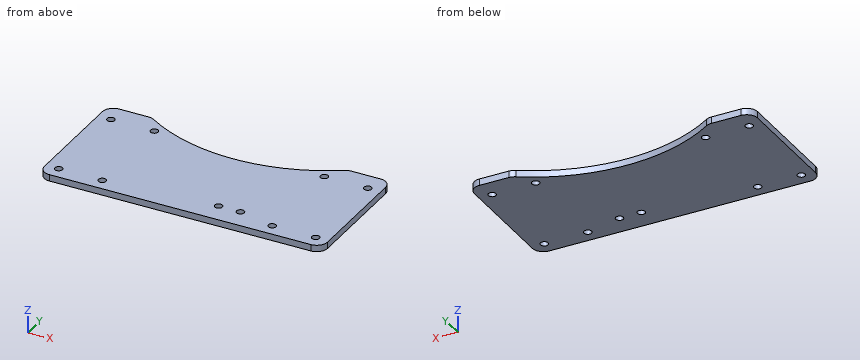
Autodesk Inventor part; units mm, degrees
ref_plane "YZ Plane" through (0, 0, 0) normal (1, 0, 0) x (0, 1, 0)
ref_plane "XZ Plane" through (0, 0, 0) normal (0, 1, 0) x (-1, 0, 0)
ref_plane "XY Plane" through (0, 0, 0) normal (0, 0, 1) x (1, 0, 0)
sketch "Sketch1" plane through (0, 0, 0) normal (0, 0, 1) x (1, 0, 0)
  line L0 (-65, -30) -> (65, -30)
  line L1 (65, -30) -> (65, 30)
  line L2 (65, 30) -> (-65, 30)
  line L3 (-65, 30) -> (-65, -30)
  line L4 (-65, -30) -> (65, 30) construction
  line L5 (65, -30) -> (-65, 30) construction
  arc A0 (-45, 30) -> (45, 30) centre (0, 96.6789) ccw
  point P0 (0, 0)
  dimension "d0" = 130
  dimension "d1" = 60
  dimension "d5" = 20
  dimension "d6" = 20
extrude "Extrusion1" add sketch "Sketch1" along normal blind 3 contours L3 L2 A0 L1 L0
fillet "Fillet1" radius 5 6 edges at (65, 30, 1.5) (65, -30, 1.5) (-65, -30, 1.5) (-65, 30, 1.5) (45, 30, 1.5) (-45, 30, 1.5)
sketch "Sketch2" plane through (0, 0, 3) normal (0, 0, 1) x (1, 0, 0)
  circle A0 centre (59, -24) radius 1.75
  circle A1 centre (39, -24) radius 1.75
  line L0 (65, -25) -> (65, 25)
  line L1 (-60, -30) -> (60, -30)
  circle A2 centre (59, 21) radius 1.75
  circle A3 centre (39, 21) radius 1.75
  line L2 (0, -30) -> (0, -45.4947)
  circle A4 centre (-59, -24) radius 1.75
  circle A5 centre (-39, -24) radius 1.75
  line L3 (-65, -25) -> (-65, 25)
  circle A6 centre (-59, 21) radius 1.75
  circle A7 centre (-39, 21) radius 1.75
  point P0 (0, 0)
  dimension "d7" = 3.5
  dimension "d8" = 3.5
  dimension "d9" = 20
  dimension "d10" = 6
  dimension "d11" = 6
  dimension "d14" = 45
extrude "Extrusion2" cut sketch "Sketch2" against normal up to surface (3 mm away)
sketch "Sketch3" plane through (0, 0, 0) normal (0, 0, -1) x (-1, 0, 0)
  circle A0 centre (-12.3926, -20.1) radius 1.75
  circle A1 centre (-22.3926, -20.1) radius 1.75
  point P0 (0, 0)
extrude "Extrusion3" cut sketch "Sketch3" against normal up to surface (3 mm away)
equation "\"d6\" = d5"
properties part number "Base plate"
The listing builds one solid part. Answer for the finished solid, in the listing's coordinates (mm). Give positions to 0.01 mm unless a question says otherwise; leave off trailing zeros. Loops run counter-clockwise (first coordinate to the right, second up) from the corner with the lowest first, then second, coordinate; pieces in that order, holes last. Notation, with made-up numbers: (-28, 4.25) - (21, 4.25) arc R23 cw to (21, 32.25) - close; hole circle Ø3 at (-16, 24). An arc over 180 degrees is marked (long way). Return JSON: item names as keys, results as strings. Group by question number.
1. Straight lines are drawn through the part: line 1 (Y direction, x = 59, z = 1); line 2 (Y direction, x = 39, z = 0.6); line 3 (X direction, y = 27.5, z = 1.1). For each, find the intervals that lie inside material, in ascending order. Write a range as [from, to].
2. Find section B-B (z = 2.3). State how many separate pieces and enclosed holes the cut face has, then the cut area to 3 significant figures.
3. Find section C-C (x = 38.5). Write down the section's boundary in (y, z), then the cut area to 3 significant figures.
4. Find section A-A (y = -20.1). Write down the section's boundary in (x, z), then the cut area to 3 significant figures.
5. Given pin 1 Ø3 at (x, y) = (-59, 21) entering from +Z; pin 2 Ø1 at (x, z) = (-4.5, 1) entering from +Y, each flat-ended and moving along its own axis, determine where each tip first touches the part or whether it passes through.
Verdict:
{
 "1": {"line 1": "y = [-30, -25.75], [-22.25, 19.25], [22.75, 30]", "line 2": "y = [-30, -25.75], [-22.25, 19.25], [22.75, 26.32]", "line 3": "x = [-64.33, -41.05], [41.05, 64.33]"},
 "2": {"separate pieces": "1", "enclosed holes": "10", "area": "6,840 mm^2"},
 "3": {"outline": "(-30, 0) - (-25.68, 0) - (-25.68, 3) - (-30, 3) - close; (-22.32, 0) - (19.32, 0) - (19.32, 3) - (-22.32, 3) - close; (22.68, 0) - (26.05, 0) - (26.05, 3) - (22.68, 3) - close", "area": "148 mm^2"},
 "4": {"outline": "(-65, 0) - (10.64, 0) - (10.64, 3) - (-65, 3) - close; (14.14, 0) - (20.64, 0) - (20.64, 3) - (14.14, 3) - close; (24.14, 0) - (65, 0) - (65, 3) - (24.14, 3) - close", "area": "369 mm^2"},
 "5": {"pin 1": "passes through", "pin 2": "stops at y = 16.39"}
}
